Part model, mm, in its own coordinate system. A direction names the side the tool comes from. Coordinates: 2 decimals unless noted, no trailing zeros. Loops run counter-clockwise (first coordinate to the right, second up) from the corner with the lowest first, then second, coordinate; pieces in that order, holes last. Notation, with made-up numbers: M 54.25,23.25 L 83.25,23.25 A24 ccw 83.25,55.25 Z; hole C 40,-35.5 d5. An arc over 180 degrees is marked long. Answer as a JSON object with one key per item and string values. Group by question number.
1. Mould opens along X. For faces 1 (the face through (-140, 63, 394)), 2 (the face through (-92, 21, -77)), 3 (the face through (-79, 0, 248)), 4 (the face through (-80, 22, 298)) say: released by +X, released by -X, zero draft, split by the parting line, or undercut.
2. Saw through at B-B on y = 58. Write the cut outline in (x, z).
3. Saw through at A-A on x = -108.5. Write the cut outline in (y, z).
4. Drop flat-ended pins along their axis: pin 1 Ø12 at (y, z) = (52, 381.5) entering from +X; pin 2 Ø10.5 at (y, z) = (20, 559.05) entering from +X; pin 3 Ø13 at (x, z) = (-130, -42.24) entering from -Y; pin 4 Ø8 at (y, z) = (23, -80.5) entering from -X. Give the stop position or say it passes through.
5. Saw through at C-C on z = 419. Write the cut outline in (x, y), then the cut area to 3 significant figures.
6. Saw through at D-D on x = 280.5. Write the cut outline in (y, z), then the cut area to 3 significant figures.
7. 3-axis set-ups, long thin cutter, end or side, ignore diameter. For faces 5 (the face through (-58, 21, -77)), 6 (the face through (-150, 63, 394)), 7 (the face through (-10, 63, 394)): which of +Z, -Z, +X, -X, +Y, -Y reach the whole face in a straight line?
8. Drill centre lines: L1, parallel to X at y = 36, z = 392.5; L2, parallel to Y at x = -109, z = -100.5; L3, parallel to X at y = 85.5, z = 395. Where is each one in solid material? Low to high.
from build123d import *

# Parameters (mm, degrees)
SKETCH2_W           = 150
SKETCH2_H           = 150
SKETCH2_R           = 4
BOSS_EXTRUDE2_DEPTH = 10
SKETCH3_W           = 10
SKETCH3_H           = 600
BOSS_EXTRUDE3_DEPTH = 45
SKETCH4_W           = 500
SKETCH4_H           = 100
BOSS_EXTRUDE4_DEPTH = 10
SKETCH5_R           = 5
BOSS_EXTRUDE5_DEPTH = 10
SKETCH7_W           = 30
SKETCH7_H           = 27
SKETCH7_R           = 4
BOSS_EXTRUDE6_DEPTH = 8.5
SKETCH8_R           = 4
CUT_EXTRUDE1_DEPTH  = 720.805795864


with BuildPart() as part:
    # Sketch2 → Boss-Extrude2 (new body)
    with BuildSketch(Plane(origin=(0, 0, 0), x_dir=(1, 0, 0), z_dir=(0, 1, 0))):
        with Locations((-75, 75)):
            Rectangle(SKETCH2_W, SKETCH2_H)
        with Locations(Location((-130, 42.241144312, 0), (0, 0, 270))):
            Circle(SKETCH2_R, mode=Mode.SUBTRACT)
        with Locations(Location((-20, 42.241144312, 0), (0, 0, 270))):
            Circle(SKETCH2_R, mode=Mode.SUBTRACT)
        with Locations(Location((-20, 107.758855688, 0), (0, 0, 90))):
            Circle(SKETCH2_R, mode=Mode.SUBTRACT)
        with Locations(Location((-130, 107.758855688, 0), (0, 0, 90))):
            Circle(SKETCH2_R, mode=Mode.SUBTRACT)
    extrude(amount=BOSS_EXTRUDE2_DEPTH)

    # Sketch3 → Boss-Extrude3 (add)
    with BuildSketch(Plane(origin=(0, 0, 0), x_dir=(1, 0, 0), z_dir=(0, 1, 0))):
        with Locations((-75, -294.045278836)):
            Rectangle(SKETCH3_W, SKETCH3_H)
    extrude(amount=BOSS_EXTRUDE3_DEPTH)

    # Sketch4 → Boss-Extrude4 (add)
    with BuildSketch(Plane(origin=(0, 0, 0), x_dir=(1, 0, 0), z_dir=(0, 1, 0))):
        with Locations((70, -394.045278836)):
            Rectangle(SKETCH4_W, SKETCH4_H)
    extrude(amount=BOSS_EXTRUDE4_DEPTH)

    # Sketch5 → Boss-Extrude5 (add)
    with BuildSketch(Plane(origin=(0, 0, 0), x_dir=(0, 0, -1), z_dir=(1, 0, 0))):
        with BuildLine():
            Line((-432.285278836, 10), (-432.285278836, 76.348788506))
            ThreePointArc((-432.285278836, 76.348788506), (-421.085042149, 103.388551818), (-394.045278836, 114.588788506))
            ThreePointArc((-394.045278836, 114.588788506), (-367.005515524, 103.388551818), (-355.805278836, 76.348788506))
            Line((-355.805278836, 76.348788506), (-355.805278836, 10))
            Line((-355.805278836, 10), (-432.285278836, 10))
        make_face()
        with Locations((-394.045278836, 76.348788506)):
            Circle(SKETCH5_R, mode=Mode.SUBTRACT)
    boss_extrude5 = extrude(amount=-BOSS_EXTRUDE5_DEPTH)

    # Mirror1: Boss-Extrude5 across plane
    add(boss_extrude5.mirror(Plane(origin=(-75, 0, 0), x_dir=(0, 0, 1), z_dir=(1, 0, 0))))

    # Sketch7 → Boss-Extrude6 (add)
    with BuildSketch(Plane(origin=(-58, 0, 0), x_dir=(0, 0, -1), z_dir=(1, 0, 0))):
        with Locations((77.164979512, 23.5)):
            Rectangle(SKETCH7_W, SKETCH7_H)
        with Locations((77.164979512, 25.524498442)):
            Circle(SKETCH7_R, mode=Mode.SUBTRACT)
    boss_extrude6 = extrude(amount=-BOSS_EXTRUDE6_DEPTH)

    # Mirror2: Boss-Extrude6 across plane
    add(boss_extrude6.mirror(Plane(origin=(-75, 0, 0), x_dir=(0, 0, 1), z_dir=(1, 0, 0))))

    # Sketch8 → Cut-Extrude1 (cut, through all)
    with BuildSketch(Plane(origin=(-70, 0, 0), x_dir=(0, 0, -1), z_dir=(1, 0, 0))):
        with Locations((-584.045278836, 20)):
            Circle(SKETCH8_R)
        with Locations((-559.045278836, 20)):
            Circle(SKETCH8_R)
    extrude(amount=-CUT_EXTRUDE1_DEPTH, mode=Mode.SUBTRACT)


solid = part.part
Outcome:
{
 "1": {"face 1": "undercut", "face 2": "released by -X", "face 3": "zero draft", "face 4": "undercut"},
 "2": {"outline": "M -150,355.81 L -140,355.81 L -140,432.29 L -150,432.29 Z; M -10,355.81 L 0,355.81 L 0,432.29 L -10,432.29 Z"},
 "3": {"outline": "M 0,-150 L 10,-150 L 10,0 L 0,0 Z; M 0,344.05 L 10,344.05 L 10,444.05 L 0,444.05 Z"},
 "4": {"pin 1": "stops at x = 0", "pin 2": "stops at x = -70", "pin 3": "stops at y = 0", "pin 4": "stops at x = -92"},
 "5": {"outline": "M -180,0 L 320,0 L 320,10 L 0,10 L 0,105.32 L -10,105.32 L -10,10 L -70,10 L -70,45 L -80,45 L -80,10 L -140,10 L -140,105.32 L -150,105.32 L -150,10 L -180,10 Z", "area": "7,260 mm²"},
 "6": {"outline": "M 0,344.05 L 10,344.05 L 10,444.05 L 0,444.05 Z", "area": "1,000 mm²"},
 "7": {"face 5": "+Z, -Z, +X, +Y", "face 6": "+Z, -Z, -X, +Y", "face 7": "+Z, -Z, +Y"},
 "8": {"L1": "x = -150 to -140, -80 to -70, -10 to 0", "L2": "y = 0 to 10", "L3": "x = -150 to -140, -10 to 0"}
}
